Source: CAD feature listing. Evaluate the final solid. Frame: model axes, mm. A direction names the side the tool comes from. Give positions to 0.01 mm unless a question says otherwise; leave off trailing zeros. Write each loop counter-clockwise with the first axis right and the second up, starting at its lowest first coordinate (ties: lowest second). Pieces come first, ordered by that corner, then holes. Notation, with made-up numbers: (17.5, 70) -> (30.5, 70) arc R24 cw to (30.5, 104) -> close; hole circle Ø11 at (-6, 53.25). An arc over 180 degrees is marked (long way). Use a Markdown table: item, result. Add a question column.
```python
from build123d import *

# Parameters (mm, degrees)
BOSS_EXTRUDE5_DEPTH     = 2
BOSS_EXTRUDE6_DEPTH     = 2
SKETCH6_R               = 11
CUT_EXTRUDE1_DEPTH      = 2
CUT_EXTRUDE3_DEPTH      = 24
CUT_EXTRUDE3_DEPTH_BACK = 35
SKETCH7_R               = 2.603714659
SKETCH8_R               = 1.4
BOSS_EXTRUDE8_DEPTH     = 4
CUT_EXTRUDE8_DEPTH      = 4
CUT_EXTRUDE9_START      = -2
SKETCH17_R              = 1.4
CUT_EXTRUDE9_DEPTH      = 2
CUT_EXTRUDE10_DEPTH     = 1
SKETCH19_R              = 3.5
CUT_EXTRUDE11_DEPTH     = 10


with BuildPart() as part:
    # Sketch1 → Boss-Extrude5 (new body)
    with BuildSketch(Plane(origin=(0, 0, 0), x_dir=(1, 0, 0), z_dir=(0, 1, 0))):
        with BuildLine():
            Line((-30, 70), (30, 70))
            ThreePointArc((30, 70), (58.284271247, 58.284271247), (70, 30))
            Line((70, 30), (70, -30))
            ThreePointArc((70, -30), (58.284271247, -58.284271247), (30, -70))
            Line((30, -70), (-30, -70))
            ThreePointArc((-30, -70), (-58.284271247, -58.284271247), (-70, -30))
            Line((-70, -30), (-70, 30))
            ThreePointArc((-70, 30), (-58.284271247, 58.284271247), (-30, 70))
        make_face()
    extrude(amount=-BOSS_EXTRUDE5_DEPTH)

    # Sketch5 → Boss-Extrude6 (add)
    with BuildSketch(Plane(origin=(0, 0, 0), x_dir=(1, 0, 0), z_dir=(0, 1, 0))):
        with BuildLine():
            Line((-28, 68), (28, 68))
            ThreePointArc((28, 68), (56.284271247, 56.284271247), (68, 28))
            Line((68, 28), (68, -28))
            ThreePointArc((68, -28), (56.284271247, -56.284271247), (28, -68))
            Line((28, -68), (-28, -68))
            ThreePointArc((-28, -68), (-56.284271247, -56.284271247), (-68, -28))
            Line((-68, -28), (-68, 28))
            ThreePointArc((-68, 28), (-56.284271247, 56.284271247), (-28, 68))
        make_face()
    extrude(amount=BOSS_EXTRUDE6_DEPTH)

    # Sketch6 → Cut-Extrude1 (cut)
    with BuildSketch(Plane.XZ.offset(2)):
        with Locations(Location((0, 0, 0), (0, 0, 270))):
            Circle(SKETCH6_R)
    extrude(amount=-CUT_EXTRUDE1_DEPTH, mode=Mode.SUBTRACT)

    # Sketch7 → Cut-Extrude3 (cut, two sides: drawn at the far end of the back side and taken through both)
    with BuildSketch(Plane.XZ.offset(-CUT_EXTRUDE3_DEPTH_BACK)):
        with Locations(Location((0, 0, 0), (0, 0, 90))):
            Circle(SKETCH7_R)
    extrude(amount=CUT_EXTRUDE3_DEPTH + CUT_EXTRUDE3_DEPTH_BACK, mode=Mode.SUBTRACT)

    # Sketch8 → Boss-Extrude8 (add)
    with BuildSketch(Plane(origin=(0, 0, 0), x_dir=(1, 0, 0), z_dir=(0, 1, 0))):
        with Locations(Location((13, 13, 0), (0, 0, 270))):
            Circle(SKETCH8_R)
        with Locations(Location((13, -13, 0), (0, 0, 270))):
            Circle(SKETCH8_R)
        with Locations(Location((-13, -13, 0), (0, 0, 270))):
            Circle(SKETCH8_R)
        with Locations(Location((-13, 13, 0), (0, 0, 270))):
            Circle(SKETCH8_R)
    extrude(amount=-BOSS_EXTRUDE8_DEPTH)

    # Sketch15 → Cut-Extrude8 (cut)
    with BuildSketch(Plane(origin=(0, 2, 0), x_dir=(1, 0, 0), z_dir=(0, 1, 0))):
        with BuildLine():
            Line((20.002895237, 8.260924079), (57.425217049, 23.761757309))
            ThreePointArc((57.425217049, 23.761757309), (60.897596895, 12.098982138), (62.152687059, -0.004839374))
            Line((62.152687059, -0.004839374), (21.647057814, -0.004839374))
            ThreePointArc((21.647057814, -0.004839374), (21.175793038, 4.197824096), (20.002895237, 8.260924079))
        make_face()
    extrude(amount=-CUT_EXTRUDE8_DEPTH, mode=Mode.SUBTRACT)

    # Sketch17 → Cut-Extrude9 (cut)
    with BuildSketch(Plane.XZ.offset(4).offset(CUT_EXTRUDE9_START)):
        with Locations((13, 13)):
            Circle(SKETCH17_R)
        with Locations((13, -13)):
            Circle(SKETCH17_R)
        with Locations((-13, -13)):
            Circle(SKETCH17_R)
        with Locations((-13, 13)):
            Circle(SKETCH17_R)
    extrude(amount=CUT_EXTRUDE9_DEPTH, mode=Mode.SUBTRACT)

    # Sketch18 → Cut-Extrude10 (cut)
    with BuildSketch(Plane.XZ.offset(2)):
        with BuildLine():
            Line((-70, 0), (-70, 4))
            Line((-70, 4), (-10.246950766, 4))
            ThreePointArc((-10.246950766, 4), (-11, 0), (-10.246950766, -4))
            Line((-10.246950766, -4), (-70, -4))
            Line((-70, -4), (-70, 0))
        make_face()
    extrude(amount=-CUT_EXTRUDE10_DEPTH, mode=Mode.SUBTRACT)

    # Sketch19 → Cut-Extrude11 (cut)
    with BuildSketch(Plane.XZ):
        with Locations(Location((0, 0, 0), (0, 0, 270))):
            Circle(SKETCH19_R)
    extrude(amount=-CUT_EXTRUDE11_DEPTH, mode=Mode.SUBTRACT)


solid = part.part
```
(1) Cut plane B-B on y = 0.8. Return the cut outline in (x, z).
(2) Mould query, pull axis X, two halves, no side actions, for faces 5 (the cylindrical face through (-56.594, 0.986, -55.972)), 6 (the flat face through (17, -2, -1)), 7 (the cylindrical face through (60.864, 0.028, -12.266)). Classes: +X half, -X half, draft (parallel to the pull), parting line (faces both ways), or undercut.
(3) Material intervals for L1, parallel to Z at x = 0, y = -1.2; L2, parallel to Y at x = -56, z = 60; L3, parallel to Z at x = 14, y = 1.35, sorted ascending.
(4) First-contact query: pin 1 Ø2 at (x, y) = (-6, 1.5) entering from +Z; pin 2 Ø0.8 at (x, y) = (-33.5, -1.5) entering from -Z; pin 3 Ø1.5 at (y, z) = (1.5, -47.5) entering from +X. Flat tips, straight axial feed; report the tip coordinate or a pass-through.
(5) Cut plane D-D on z = -41. Return the cut outline in (x, y), then the cut area to 3 significant figures.
(6) Cut plane C-C on x = -23. Return the cut outline in (y, z), then the cut area to 3 significant figures.
(7) Access query for faces 1 (the cylindrical face through (21.187, 0.028, -4.14)), 2 (the cylindrical face through (9.275, -1.014, -5.914)), 3 (the cylindrical face through (55.972, 0.986, -56.594)), 4 (the cylindrical face through (56.594, 0.986, 55.972)). Directions: +Z, -Z, +X, -X, +Y, -Y. A direction counts if a zero-diameter tool reaches every point of the face in a straight line with its end or side. Return the directions, or none.
(8) Cut plane A-A on x = 0. Return the cut outline in (y, z), then the cut area to 3 significant figures.
Output:
| question | item | result |
|---|---|---|
| 1 | outline | (-68, -28) arc R40 ccw to (-28, -68) -> (28, -68) arc R40 ccw to (68, -28) -> (68, 28) arc R40 ccw to (28, 68) -> (-28, 68) arc R40 ccw to (-68, 28) -> close; hole circle Ø7 at (0, 0); hole (20, -8.26) -> (57.43, -23.76) arc R65.5 ccw to (62.15, 0) -> (21.65, 0) arc R25 cw to start |
| 2 | face 5 | -X half |
| 2 | face 6 | draft |
| 2 | face 7 | undercut |
| 3 | L1 | -70 to -11, 11 to 70 |
| 3 | L2 | -2 to 0 |
| 3 | L3 | -68 to 68 |
| 4 | pin 1 | z = 68 |
| 4 | pin 2 | z = -69.88 |
| 4 | pin 3 | x = 63.33 |
| 5 | outline | (-68.46, -2) -> (68.46, -2) -> (68.46, 0) -> (65.83, 0) -> (65.83, 2) -> (-65.83, 2) -> (-65.83, 0) -> (-68.46, 0) -> close |
| 5 | area | 537 mm^2 |
| 6 | outline | (-2, -70) -> (0, -70) -> (0, -68) -> (2, -68) -> (2, 68) -> (0, 68) -> (0, 70) -> (-2, 70) -> (-2, 4) -> (-1, 4) -> (-1, -4) -> (-2, -4) -> close |
| 6 | area | 544 mm^2 |
| 7 | face 1 | +Y, -Y |
| 7 | face 2 | -Y |
| 7 | face 3 | -Z, +X, +Y |
| 7 | face 4 | +Z, +X, +Y |
| 8 | outline | (-2, -70) -> (0, -70) -> (0, -68) -> (2, -68) -> (2, -3.5) -> (0, -3.5) -> (0, -11) -> (-2, -11) -> close; (-2, 11) -> (0, 11) -> (0, 3.5) -> (2, 3.5) -> (2, 68) -> (0, 68) -> (0, 70) -> (-2, 70) -> close |
| 8 | area | 494 mm^2 |
